from build123d import *

# Parameters (mm, degrees)
SKETCH1_W           = 88.9
SKETCH1_H           = 63.5
BOSS_EXTRUDE1_DEPTH = 15.24
BOSS_EXTRUDE2_DEPTH = 63.5
CUT_EXTRUDE1_DEPTH  = 63.5


with BuildPart() as part:
    # Sketch1 → Boss-Extrude1 (new body)
    with BuildSketch(Plane(origin=(0, 0, 0), x_dir=(1, 0, 0), z_dir=(0, 1, 0))):
        Rectangle(SKETCH1_W, SKETCH1_H)
    extrude(amount=BOSS_EXTRUDE1_DEPTH)

    # Sketch2 → Boss-Extrude2 (add)
    with BuildSketch(Plane.XY.offset(31.75)):
        Polygon((44.45, 15.24), (59.69, 0), (44.45, 0), align=None)
    extrude(amount=-BOSS_EXTRUDE2_DEPTH)

    # Sketch3 → Cut-Extrude1 (cut)
    with BuildSketch(Plane(origin=(0, 0, -31.75), x_dir=(-1, 0, 0), z_dir=(0, 0, -1))):
        Polygon((44.45, 15.24), (29.21, 0), (44.45, 0), align=None)
    extrude(amount=-CUT_EXTRUDE1_DEPTH, mode=Mode.SUBTRACT)


solid = part.part
Input: part model. Units: mm. Frame: model coordinates. Round coordinates to 2 decimals unless told otherwise and drop trailing zeros. Loops run counter-clockwise (first coordinate to the right, second up) from the corner with the lowest first, then second, coordinate; pieces in that order, holes last. Notation, with made-up numbers: M 30.5,-31 L 80.5,-31 A8 ccw 80.5,-22 Z; hole C 56.5,1.25 d5. An arc over 180 degrees is marked long. Answer as CSV lines item,"result". Start each with the question number.
(1) Section A-A, the plane y = 14.25. Output: boundary loops of the cut face in (x, z), plus the area to 3 significant figures.
(2) Section B-B, the plane z = -1. Output: boundary loops of the cut face in (x, y), plus the area to 3 significant figures.
(3) First-contact query: pin 1 (4 mm diameter, centred on y = 7, z = 14.5, fed in from -X); pin 2 (5 mm diameter, centred on y = 12, z = 1, fed in from -X); pin 3 (5 mm diameter, centred on y = 6.5, z = 18.5, fed in from +X). Flat tips, straight axial feed; report the tip coordinate or a pass-through.
(4) Line query: line 1 (Y direction, x = -40, z = 10); line 2 (X direction, y = 4.5, z = -25.5); line 3 (X direction, y = 14, z = -2.5). Output: solid intervals per line, ascending. Write a range as [from, to].
Values found:
1,outline,"M -43.46,-31.75 L 45.44,-31.75 L 45.44,31.75 L -43.46,31.75 Z"
1,area,"5,650 mm²"
2,outline,"M -44.45,15.24 L -29.21,0 L 59.69,0 L 44.45,15.24 Z"
2,area,"1,350 mm²"
3,pin 1,"stops at x = -38.21"
3,pin 2,"stops at x = -43.71"
3,pin 3,"stops at x = 55.69"
4,line 1,"y = [10.79, 15.24]"
4,line 2,"x = [-33.71, 55.19]"
4,line 3,"x = [-43.21, 45.69]"
